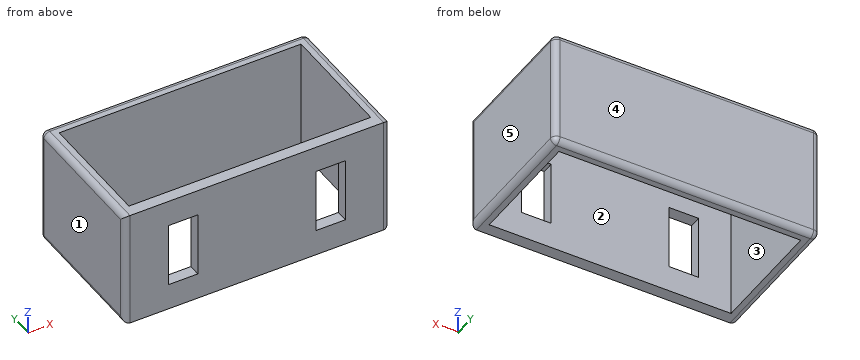
```python
from build123d import *

# Parameters (mm, degrees)
F0_W     = 45
F0_H     = 20
F1_DEPTH = 24
F2_W     = 41
F2_H     = 20
F3_DEPTH = 20
F5_W     = 5
F5_H     = 11
F6_DEPTH = 5
F7_R     = 1


with BuildPart() as f1:
    # F0 (on Front) → F1 (new body)
    with BuildSketch(Plane.XZ):
        with Locations((22.5, -10)):
            Rectangle(F0_W, F0_H)
    extrude(amount=F1_DEPTH)

    # F2 (on Top) → F3 (cut, symmetric)
    with BuildSketch(Plane.XY):
        with Locations((22.5, -12)):
            Rectangle(F2_W, F2_H)
    extrude(amount=F3_DEPTH, both=True, mode=Mode.SUBTRACT)

    # F5 (on offset) → F6 (cut)
    with BuildSketch(Plane(origin=(0, -22, 0), x_dir=(-1, 0, 0), z_dir=(0, 1, 0))):
        with Locations((-10, -10)):
            Rectangle(F5_W, F5_H)
        with Locations((-35, -9.9999997467)):
            Rectangle(F5_W, F5_H)
    extrude(amount=-F6_DEPTH, mode=Mode.SUBTRACT)

    # F7
    f7_edges = [f1.edges().sort_by_distance(p)[0] for p in [
        (45, -12, -20),
        (45, -12, 0),
        (45, 0, -10),
        (45, -24, -10),
        (22.5, 0, 0),
        (0, 0, -10),
        (22.5, 0, -20),
        (0, -12, 0),
        (0, -12, -20),
        (0, -24, -10),
    ]]
    fillet(f7_edges, radius=F7_R)


solid = f1.part
```
Can you work these out from the model? Positions are in its coordinate system, mm. Face numbers are marked on the shaded views. A direction names the side the tool comes from. Coordinates: 2 decimals unless noted, no trailing zeros. Loops run counter-clockwise (first coordinate to the right, second up) from the corner with the lowest first, then second, coordinate; pieces in that order, holes last. Notation, with made-up numbers: (81, -11.5) - (91, -11.5) arc R24 cw to (91, 13.5) - close; hole circle Ø6 at (5.5, 46). An arc over 180 degrees is marked (long way). Use a Markdown table: item, result.
Item 1: I want a section at B-B on x = 34.5. Please give me the cut outline in (y, z), and give its area (3 significant figures).
Numbers:
| item | result |
|---|---|
| outline | (-24, -20) - (-22, -20) - (-22, -15.5) - (-24, -15.5) - close; (-24, -4.5) - (-22, -4.5) - (-22, 0) - (-24, 0) - close; (-2, -20) - (-1, -20) arc R1 ccw to (0, -19) - (0, -1) arc R1 ccw to (-1, 0) - (-2, 0) - close |
| area | 57.6 mm2 |
Item 2: Will this pin go through, and if not, where does the flat tip stop? pin 1 (1 mm diameter, centred on x = 23, y = -20.5, fed in from -Z).
Numbers:
| item | result |
|---|---|
| pin 1 | passes through |
Item 3: I want a section at D-D on y = -8.5. Please give me the cut outline in (x, z), and give its area (3 significant figures).
Numbers:
| item | result |
|---|---|
| outline | (0, -19) arc R1 ccw to (1, -20) - (2, -20) - (2, 0) - (1, 0) arc R1 ccw to (0, -1) - close; (43, -20) - (44, -20) arc R1 ccw to (45, -19) - (45, -1) arc R1 ccw to (44, 0) - (43, 0) - close |
| area | 79.1 mm2 |
Item 4: We'd pull the mould along X, two halves only. Please class the marked faces 3, 4 and 5: released by +X, released by -X, zero draft, split by the parting line, or undercut.
Numbers:
| item | result |
|---|---|
| face 3 | undercut |
| face 4 | zero draft |
| face 5 | released by +X |
Item 5: If I drill on probe 1 along X at (y, z) = (-22.25, -13.5); probe 2 along X at (y, z) = (-21.5, -9.25); probe 3 along Y at (x, z) = (22.5, -8), over which ranges is the centre line in solid material (lowest first)? Write a range as from..to.
Numbers:
| item | result |
|---|---|
| probe 1 | x = 0..7.5, 12.5..32.5, 37.5..45 |
| probe 2 | x = 0..2, 43..45 |
| probe 3 | y = -24..-22, -2..0 |
Item 6: I want a section at A-A on z = -12. Please give me the cut outline in (x, y).
Numbers:
| item | result |
|---|---|
| outline | (0, -23) arc R1 ccw to (1, -24) - (7.5, -24) - (7.5, -22) - (2, -22) - (2, -2) - (43, -2) - (43, -22) - (37.5, -22) - (37.5, -24) - (44, -24) arc R1 ccw to (45, -23) - (45, -1) arc R1 ccw to (44, 0) - (1, 0) arc R1 ccw to (0, -1) - close; (12.5, -24) - (32.5, -24) - (32.5, -22) - (12.5, -22) - close |
Item 7: For the marked faces 1 and 2, which set-ups out of +Z, -Z, +X, -X, +Y, -Y let a thin tool reach every point of the face, with its end or its side?
Numbers:
| item | result |
|---|---|
| face 1 | +Z, -Z, -X, +Y, -Y |
| face 2 | +Z, -Z |
Item 8: I want a section at C-C on z = -2.75. Please give me the cut outline in (x, y), and give its area (3 significant figures).
Numbers:
| item | result |
|---|---|
| outline | (0, -23) arc R1 ccw to (1, -24) - (44, -24) arc R1 ccw to (45, -23) - (45, -1) arc R1 ccw to (44, 0) - (1, 0) arc R1 ccw to (0, -1) - close; hole (2, -22) - (43, -22) - (43, -2) - (2, -2) - close |
| area | 259 mm2 |
